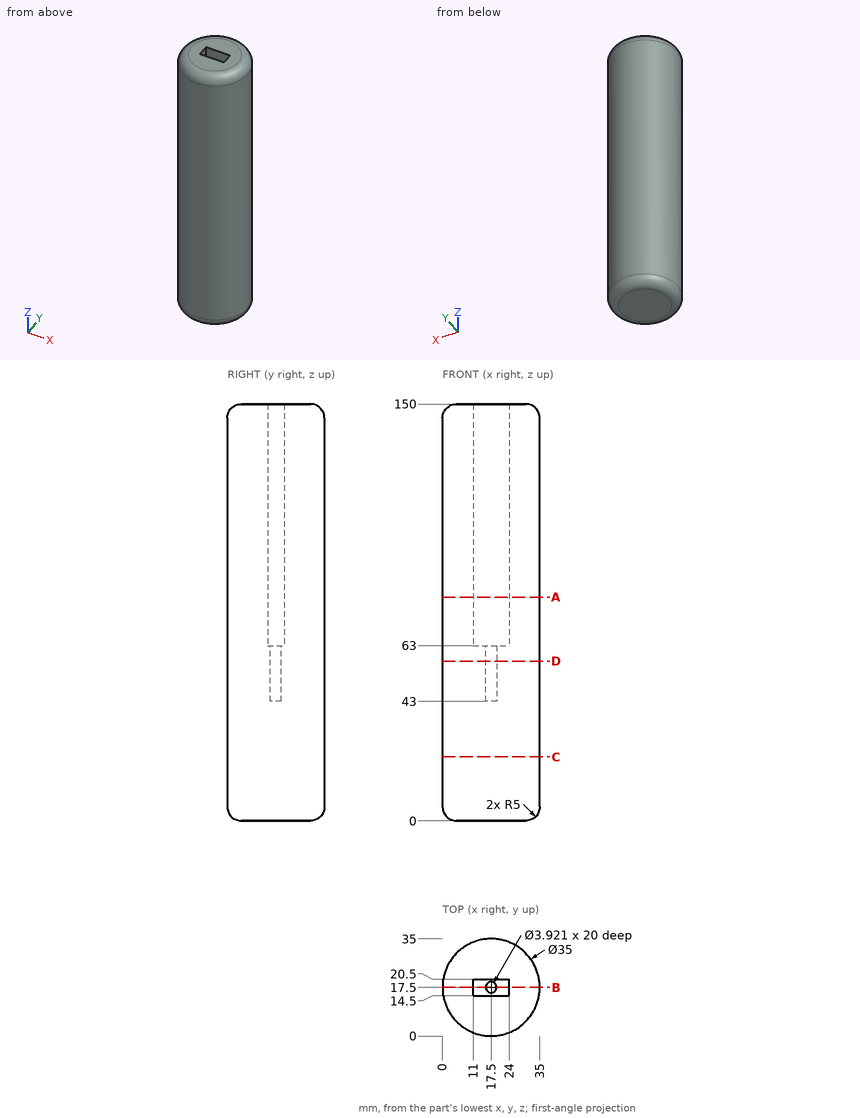
Geometry: see drawing. Coordinates: mm, zero at the bounding-box minimum. Give positions to 0.01 mm unless a question says otherwise; leave off trailing zeros. Write each loop counter-clockwise with the first axis right and the second up, starting at its lowest first coordinate (ties: lowest second). Pieces come first, ordered by that corner, then holes. Notation, with made-up numbers: (-6.75, 82.25) - (30.25, 82.25) arc R19 ccw to (30.25, 105.25) - close; hole circle Ø3 at (9.25, 8.5). An arc over 180 degrees is marked (long way). Return JSON: item names as keys, results as strings. Group by question number.
1) Section C-C on z = 23. Return the cut outline in (x, y), plus the area to 3 significant figures.
2) Section B-B on y = 17.5. Return the cut outline in (x, z), plus the area to 3 significant figures.
3) Line query: line 1 (Y direction, x = 17.5, z = 55.75); line 2 (Y direction, x = 18, z = 97); line 3 (X direction, y = 18.5, z = 74.5). Output: solid intervals per line, ascending.
4) Section A-A on z = 80.5. Return the cut outline in (x, y), plus the area to 3 significant figures.
5) Section D-D on z = 57.5. Return the cut outline in (x, y).
6) First-contact query: P1, Ø2, axis at x = 7.5, z = 47, coming from the -Y side; P2, Ø4.5, axis at x = 17.5, y = 18, coming from the +Z side; P3, Ø2, axis at x = 25.5, z = 75, coming from the +Y side. Flat tips, straight axial feed; report the tip coordinate or a pass-through.
Filled in:
{
 "1": {"outline": "circle Ø35 at (17.5, 17.5)", "area": "962 mm^2"},
 "2": {"outline": "(0, 5) arc R5 ccw to (5, 0) - (30, 0) arc R5 ccw to (35, 5) - (35, 145) arc R5 ccw to (30, 150) - (24, 150) - (24, 63) - (19.46, 63) - (19.46, 43) - (15.54, 43) - (15.54, 63) - (11, 63) - (11, 150) - (5, 150) arc R5 ccw to (0, 145) - close", "area": "4,020 mm^2"},
 "3": {"line 1": "y = 0 to 15.54, 19.46 to 35", "line 2": "y = 0.01 to 14.5, 20.5 to 34.99", "line 3": "x = 0.03 to 11, 24 to 34.97"},
 "4": {"outline": "circle Ø35 at (17.5, 17.5); hole (11, 14.5) - (24, 14.5) - (24, 20.5) - (11, 20.5) - close", "area": "884 mm^2"},
 "5": {"outline": "circle Ø35 at (17.5, 17.5); hole circle Ø3.92 at (17.5, 17.5)"},
 "6": {"P1": "stops at y = 2.49", "P2": "stops at z = 63", "P3": "stops at y = 33.54"}
}
